The listing builds one solid part. Answer for the finished solid, in the listing's coordinates (mm). Coordinates: 2 decimals unless noted, no trailing zeros. Answer as a JSON object with one key per item and string values. Group by question number.
1. Straight lines are drawn through the part: L1, parallel to Y at x = 618.5, z = 8.25; L2, parallel to Y at x = 413.5, z = 4.75; L3, parallel to Y at x = 11, z = 7.5. For each, find the intervals that lie inside material, in ascending order.
2. Determine the mould class of faces 1 (the face through (308, 0, 7)), 2 (the face through (308, 120, 7)), 3 (the face through (625, 59, 12)) for opening direction Y: released by +Y, released by -Y, zero draft, split by the parting line, or undercut.
3. A cutting plane is placed at A-A on z = 7. State how many separate pieces and enclosed holes the cut face has, and give its area (3 significant figures).
4. Given pin 1 (5 mm diameter, centred on y = 60, z = 7.5, fed in from -X); pin 2 (5 mm diameter, centred on x = 618.5, y = 7.5, fed in from +Z), each flat-ended and moving along its own axis, determine where each tip first touches the part or whether it passes through.
from build123d import *

# Parameters (mm, degrees)
ESQUISSE1_W                  = 625
ESQUISSE1_H                  = 120
BOSS_EXTRU_1_DEPTH           = 15
ENL_V_MAT_EXTRU_1_DEPTH      = 637.592491316
ENL_V_MAT_EXTRU_1_DEPTH_BACK = 637.592491316
ESQUISSE2_R                  = 2.75
CONG_1_R                     = 5
ESQUISSE3_R                  = 4.1
ENL_V_MAT_EXTRU_2_DEPTH      = 20
ENL_V_START                  = -605
ESQUISSE3_2_R                = 4.1
ENL_V_MAT_EXTRU_3_DEPTH      = 20
ENL_V_MAT_EXTRU_4_DEPTH      = 637.592491316
ENL_V_MAT_EXTRU_4_DEPTH_BACK = 637.592491316
ESQUISSE4_R                  = 2.5


with BuildPart() as part:
    # Esquisse1 → Boss.-Extru.1 (new body)
    with BuildSketch(Plane.XY):
        with Locations((312.5, 60)):
            Rectangle(ESQUISSE1_W, ESQUISSE1_H)
    extrude(amount=BOSS_EXTRU_1_DEPTH)

    # Esquisse2 → Enlèv. mat.-Extru.1 (cut, two sides: drawn at the far end of the back side and taken through both)
    with BuildSketch(Plane.XY.offset(15).offset(-ENL_V_MAT_EXTRU_1_DEPTH_BACK)):
        with Locations((6.5, 112.5)):
            Circle(ESQUISSE2_R)
        with Locations((6.5, 82.5)):
            Circle(ESQUISSE2_R)
        with Locations(Location((38.5, 82.5, 0), (0, 0, 180))):
            Circle(ESQUISSE2_R)
        with Locations(Location((38.5, 112.5, 0), (0, 0, 180))):
            Circle(ESQUISSE2_R)
        with Locations((38.5, 7.5)):
            Circle(ESQUISSE2_R)
        with Locations((38.5, 37.5)):
            Circle(ESQUISSE2_R)
        with Locations(Location((6.5, 37.5, 0), (0, 0, 180))):
            Circle(ESQUISSE2_R)
        with Locations(Location((6.5, 7.5, 0), (0, 0, 180))):
            Circle(ESQUISSE2_R)
        with Locations((618.5, 7.5)):
            Circle(ESQUISSE2_R)
        with Locations((618.5, 37.5)):
            Circle(ESQUISSE2_R)
        with Locations(Location((586.5, 37.5, 0), (0, 0, 180))):
            Circle(ESQUISSE2_R)
        with Locations(Location((586.5, 7.5, 0), (0, 0, 180))):
            Circle(ESQUISSE2_R)
        with Locations((586.5, 112.5)):
            Circle(ESQUISSE2_R)
        with Locations((586.5, 82.5)):
            Circle(ESQUISSE2_R)
        with Locations(Location((618.5, 82.5, 0), (0, 0, 180))):
            Circle(ESQUISSE2_R)
        with Locations(Location((618.5, 112.5, 0), (0, 0, 180))):
            Circle(ESQUISSE2_R)
    extrude(amount=ENL_V_MAT_EXTRU_1_DEPTH + ENL_V_MAT_EXTRU_1_DEPTH_BACK, mode=Mode.SUBTRACT)

    # Congé1
    cong_1_edges = [part.edges().sort_by_distance(p)[0] for p in [
        (0, 120, 7.5),
        (625, 120, 7.5),
        (625, 0, 7.5),
        (0, 0, 7.5),
    ]]
    fillet(cong_1_edges, radius=CONG_1_R)

    # Esquisse3 → Enlèv. mat.-Extru.2 (cut)
    with BuildSketch(Plane(origin=(625, 0, 0), x_dir=(0, 0, -1), z_dir=(1, 0, 0))):
        with Locations((-7.5, 60)):
            Circle(ESQUISSE3_R)
    extrude(amount=-ENL_V_MAT_EXTRU_2_DEPTH, mode=Mode.SUBTRACT)

    # Esquisse3<2> → Enlèv. mat.-Extru.3 (cut)
    with BuildSketch(Plane(origin=(625, 0, 0), x_dir=(0, 0, -1), z_dir=(1, 0, 0)).offset(ENL_V_START)):
        with Locations((-7.5, 60)):
            Circle(ESQUISSE3_2_R)
    extrude(amount=-ENL_V_MAT_EXTRU_3_DEPTH, mode=Mode.SUBTRACT)

    # Esquisse4 → Enlèv. mat.-Extru.4 (cut, two sides: drawn at the far end of the back side and taken through both)
    with BuildSketch(Plane.XY.offset(15).offset(-ENL_V_MAT_EXTRU_4_DEPTH_BACK)):
        with Locations((265.5, 80)):
            Circle(ESQUISSE4_R)
        with Locations(Location((285.5, 80, 0), (0, 0, 180))):
            Circle(ESQUISSE4_R)
        with Locations((285.5, 40)):
            Circle(ESQUISSE4_R)
        with Locations(Location((265.5, 40, 0), (0, 0, 180))):
            Circle(ESQUISSE4_R)
        with Locations((359.5, 40)):
            Circle(ESQUISSE4_R)
        with Locations(Location((339.5, 40, 0), (0, 0, 180))):
            Circle(ESQUISSE4_R)
        with Locations((339.5, 80)):
            Circle(ESQUISSE4_R)
        with Locations(Location((359.5, 80, 0), (0, 0, 180))):
            Circle(ESQUISSE4_R)
        with Locations((211.5, 40)):
            Circle(ESQUISSE4_R)
        with Locations(Location((191.5, 40, 0), (0, 0, 180))):
            Circle(ESQUISSE4_R)
        with Locations((191.5, 80)):
            Circle(ESQUISSE4_R)
        with Locations(Location((211.5, 80, 0), (0, 0, 180))):
            Circle(ESQUISSE4_R)
        with Locations((117.5, 80)):
            Circle(ESQUISSE4_R)
        with Locations(Location((137.5, 80, 0), (0, 0, 180))):
            Circle(ESQUISSE4_R)
        with Locations((137.5, 40)):
            Circle(ESQUISSE4_R)
        with Locations(Location((117.5, 40, 0), (0, 0, 180))):
            Circle(ESQUISSE4_R)
        with Locations((507.5, 40)):
            Circle(ESQUISSE4_R)
        with Locations(Location((487.5, 40, 0), (0, 0, 180))):
            Circle(ESQUISSE4_R)
        with Locations((487.5, 80)):
            Circle(ESQUISSE4_R)
        with Locations(Location((507.5, 80, 0), (0, 0, 180))):
            Circle(ESQUISSE4_R)
        with Locations((413.5, 80)):
            Circle(ESQUISSE4_R)
        with Locations(Location((433.5, 80, 0), (0, 0, 180))):
            Circle(ESQUISSE4_R)
        with Locations((433.5, 40)):
            Circle(ESQUISSE4_R)
        with Locations(Location((413.5, 40, 0), (0, 0, 180))):
            Circle(ESQUISSE4_R)
    extrude(amount=ENL_V_MAT_EXTRU_4_DEPTH + ENL_V_MAT_EXTRU_4_DEPTH_BACK, mode=Mode.SUBTRACT)


solid = part.part
From the geometry:
{
 "1": {"L1": "y = 0 to 4.75, 10.25 to 34.75, 40.25 to 55.97, 64.03 to 79.75, 85.25 to 109.75, 115.25 to 120", "L2": "y = 0 to 37.5, 42.5 to 77.5, 82.5 to 120", "L3": "y = 0 to 55.9, 64.1 to 120"},
 "2": {"face 1": "released by -Y", "face 2": "released by +Y", "face 3": "zero draft"},
 "3": {"separate pieces": "1", "enclosed holes": "40", "area": "73,800 mm²"},
 "4": {"pin 1": "stops at x = 20", "pin 2": "passes through"}
}
